```python
from build123d import *

# Parameters (mm, degrees)
SKETCH1_W           = 26
SKETCH1_H           = 22
SKETCH1_W_2         = 22
SKETCH1_H_2         = 18
BOSS_EXTRUDE1_DEPTH = 2
SKETCH1_3_W         = 26
SKETCH1_3_H         = 22
SKETCH1_3_W_2       = 22
SKETCH1_3_H_2       = 18
BOSS_EXTRUDE2_DEPTH = 12.5
SKETCH2_W           = 2
SKETCH2_H           = 10
SKETCH2_H_2         = 7.5
CUT_EXTRUDE1_DEPTH  = 10.5


with BuildPart() as part:
    # Sketch1 → Boss-Extrude1 (new body)
    # profile 1 of 2: a face of its own
    with BuildSketch(Plane(origin=(0, 0, 0), x_dir=(1, 0, 0), z_dir=(0, 1, 0))):
        with Locations((11, 9)):
            Rectangle(SKETCH1_W, SKETCH1_H)
        with Locations((11, 9)):
            Rectangle(SKETCH1_W_2, SKETCH1_H_2, mode=Mode.SUBTRACT)
    # profile 2 of 2: a face of its own
    with BuildSketch(Plane(origin=(0, 0, 0), x_dir=(1, 0, 0), z_dir=(0, 1, 0))):
        with Locations((11, 9)):
            Rectangle(SKETCH1_W_2, SKETCH1_H_2)
    extrude(amount=BOSS_EXTRUDE1_DEPTH)

    # Sketch1<3> → Boss-Extrude2 (add)
    with BuildSketch(Plane(origin=(0, 0, 0), x_dir=(1, 0, 0), z_dir=(0, 1, 0))):
        with Locations((11, 9)):
            Rectangle(SKETCH1_3_W, SKETCH1_3_H)
        with Locations((11, 9)):
            Rectangle(SKETCH1_3_W_2, SKETCH1_3_H_2, mode=Mode.SUBTRACT)
    extrude(amount=BOSS_EXTRUDE2_DEPTH)

    # Sketch2 → Cut-Extrude1 (cut)
    with BuildSketch(Plane(origin=(0, 12.5, 0), x_dir=(1, 0, 0), z_dir=(0, 1, 0))):
        with Locations((-1, 5)):
            Rectangle(SKETCH2_W, SKETCH2_H)
        with Locations((23, 3.75)):
            Rectangle(SKETCH2_W, SKETCH2_H_2)
    extrude(amount=-CUT_EXTRUDE1_DEPTH, mode=Mode.SUBTRACT)


solid = part.part
```
Can you work these out from the model? Positions are in its coordinate system, mm. A direction names the side the tool comes from. Coordinates: 2 decimals unless noted, no trailing zeros. Loops run counter-clockwise (first coordinate to the right, second up) from the corner with the lowest first, then second, coordinate; pieces in that order, holes last. Notation, with made-up numbers: (-10, 31.5) - (-2, 31.5) arc R28 ccw to (-2, 57.5) - close; hole circle Ø11 at (52.25, 4.5). An arc over 180 degrees is marked (long way). Use a Markdown table: item, result.
Item 1: I want a section at A-A on y = 3.5. Please give me the cut outline in (x, z).
Numbers:
| item | result |
|---|---|
| outline | (-2, -20) - (24, -20) - (24, -7.5) - (22, -7.5) - (22, -18) - (0, -18) - (0, -10) - (-2, -10) - close; (-2, 0) - (24, 0) - (24, 2) - (-2, 2) - close |
Item 2: For faces 1 (the face through (11, 7, 0)), 2 (the face through (11, 7, -18)), 3 (the face through (-1, 7, -10)), 4 (the face through (11, 6, -20)), which set-ups out of +Z, -Z, +X, -X, +Y, -Y let a thin tool reach every point of the face, with its end or its side?
Numbers:
| item | result |
|---|---|
| face 1 | +X, -X, +Y |
| face 2 | +Y |
| face 3 | -X, +Y |
| face 4 | -Z, +X, -X, +Y, -Y |
Item 3: I want a section at B-B on z = -14.5. Please give me the cut outline in (x, y).
Numbers:
| item | result |
|---|---|
| outline | (-2, 0) - (24, 0) - (24, 12.5) - (22, 12.5) - (22, 2) - (0, 2) - (0, 12.5) - (-2, 12.5) - close |
Item 4: I want a section at D-D on z = -9. Please give me the cut outline in (x, y).
Numbers:
| item | result |
|---|---|
| outline | (-2, 0) - (24, 0) - (24, 12.5) - (22, 12.5) - (22, 2) - (-2, 2) - close |
Item 5: If I drill on probe 1 along Z at (x, y) = (3.5, 6.25); probe 2 along X at (y, z) = (10.5, -10.25); probe 3 along Z at (x, y) = (22.25, 4.5), over which ranges is the centre line in solid material (lowest first)? Write a range as from..to.
Numbers:
| item | result |
|---|---|
| probe 1 | z = -20..-18, 0..2 |
| probe 2 | x = -2..0, 22..24 |
| probe 3 | z = -20..-7.5, 0..2 |
Item 6: We'd pull the mould along X, two halves only. Please class faces 5 (the face through (22, 7, -13)), 6 (the face through (24, 6, -11)), 7 (the face through (-2, 5, -11)): released by +X, released by -X, zero draft, split by the parting line, or undercut.
Numbers:
| item | result |
|---|---|
| face 5 | undercut |
| face 6 | released by +X |
| face 7 | released by -X |
Item 7: I want a section at C-C on x = 6. Please give me the cut outline in (y, z).
Numbers:
| item | result |
|---|---|
| outline | (0, -20) - (12.5, -20) - (12.5, -18) - (2, -18) - (2, 0) - (12.5, 0) - (12.5, 2) - (0, 2) - close |
Item 8: Will this pin go through, and if not, where does the flat tip stop? pin 1 (5.5 mm diameter, centred on x = 10.5, z = -7.5, fed in from +Y).
Numbers:
| item | result |
|---|---|
| pin 1 | stops at y = 2 |
